Autodesk Inventor part; units mm, degrees
ref_plane "Work Plane1" through (25.5, 0, 0) normal (1, 0, 0) x (0, 0, -1)
ref_plane "Work Plane2" through (17.5, 0, 0) normal (-1, 0, 0) x (0, 0, 1)
ref_plane "YZ Plane" through (0, 0, 0) normal (1, 0, 0) x (0, 1, 0)
sketch "Sketch1" plane through (0, 0, 0) normal (1, 0, 0) x (0, 1, 0)
  circle A0 centre (0, 0) radius 2.85
  dimension "diameter" = 5.7
extrude "Shaft" add sketch "Sketch1" along normal mid plane 47
sketch "Sketch2" plane through (0, 0, 0) normal (0, 0, 1) x (1, 0, 0)
  line L0 (-23.5, -2.85) -> (-23.5, 2.85) construction
  line L1 (23.5, -2.85) -> (-23.5, -2.85) construction
  line L2 (23.5, 2.85) -> (23.5, -2.85) construction
  line L3 (-23.5, 2.85) -> (23.5, 2.85) construction
  line L4 (-23.5, -2.85) -> (23.5, -2.85)
  line L5 (-16.5, -2.85) -> (-16.5, -2.85)
  line L6 (-23.5, -2.85) -> (23.5, -2.85)
  line L7 (-21.5, 0) -> (-17.5, 0) construction
  line L8 (-20.6, -0.9) -> (-18.4, -0.9)
  line L9 (-18.4, 0.9) -> (-20.6, 0.9)
  arc A0 (-20.6, 0.9) -> (-20.6, -0.9) centre (-20.6, 0) ccw
  arc A1 (-18.4, -0.9) -> (-18.4, 0.9) centre (-18.4, 0) ccw
  point P0 (0, 0)
  point P1 (23.5, 0)
  point P2 (-19.5, 0)
  dimension "d17" = 1.8
  dimension "d20" = 2
  dimension "d21" = 1
  dimension "d22" = 7
extrude "Slot for Differential Gear" cut sketch "Sketch2" along normal through all both and the other way through all
ref_plane "Work Plane1" through (25.5, 0, 0) normal (1, 0, 0) x (0, 0, -1)
sketch "Sketch3" plane through (25.5, 0, 0) normal (1, 0, 0) x (0, 0, -1)
  arc A0 (1.6583, -2.5) -> (-1.6583, -2.5) centre (0, 0) ccw construction
  circle A1 centre (0, 0) radius 2.85 construction
  line L0 (-1.6583, -2.5) -> (1.6583, -2.5)
  arc A2 (1.6125, -2.35) -> (-1.6125, -2.35) centre (0, 0) ccw
  line L1 (1.6125, -2.35) -> (-1.6125, -2.35)
  point P0 (-1.3684, -2.5)
  point P1 (1.3684, -2.5)
  dimension "d49" = 3
  dimension "d50" = 2.5
  dimension "wheel_offset" = 0.15
extrude "Wheel Insert Profile" add sketch "Sketch3" along normal blind 12
loft "Loft1" add section 1 edges at (23.5, -2.85, 0) section 2 edges at (25.5, -2.35, 0) (25.5, 2.85, 0)
ref_plane "Work Plane2" through (17.5, 0, 0) normal (-1, 0, 0) x (0, 0, 1)
sketch "Sketch4" plane through (17.5, 0, 0) normal (-1, 0, 0) x (0, 0, 1)
  circle A0 centre (0, 0) radius 3.75
  dimension "d35" = 7.5
extrude "Stopper" add sketch "Sketch4" against normal blind 1
fillet "Fillet1" radius 0.5 2 edges at (17.5, 0, -3.75) (18.5, 0, -3.75)
sketch "Sketch8" plane through (-23.5, 0, 0) normal (-1, 0, 0) x (0, 0, 1)
  circle A0 centre (0, 0) radius 2.85
  circle A1 centre (0, 0) radius 2.7 construction
  circle A2 centre (0, 0) radius 2.65
  dimension "d68" = 5.4
  dimension "d69" = 0.05
extrude "Differential Gear Insert Profile" cut sketch "Sketch8" against normal blind 8
fillet "Fillet3" radius 1 1 edges at (-15.5, -2.85, 0)
chamfer "Chamfer4" distance 0.5 angle 45 2 edges at (-23.5, 0, -2.65) (37.5, 2.85, 0)
properties part number "rear shaft v2"
The listing builds one solid part. Answer for the finished solid, in the listing's coordinates (mm). A direction names the side the tool comes from. Round coordinates to 2 decimals unless told otherwise and drop trailing zeros. Write each loop counter-clockwise with the first axis right and the second up, starting at its lowest first coordinate (ties: lowest second). Pieces come first, ordered by that corner, then holes. Notation, with made-up numbers: M 87.5,25 L 103.5,25 A7 cw 103.5,29 Z; hole C 78.5,-37 d7. An arc over 180 degrees is marked long. Write each question's results on one line, items separated by ' | '. Start each with the question number.
(1) Determine the mould class of faces 1 (the cylindrical face through (-17.5, 0, 0)), 2 (the cylindrical face through (31.17, 2.85, 0.1)), 3 (the flat face through (-23.5, 0, 0)) for opening direction Y: +Y half, -Y half, draft (parallel to the pull), parting line (faces both ways), or undercut.
(2) Find the intervals of material crossed by line 1 (X direction, y = -0.25, z = -2.25); line 2 (X direction, y = 2.25, z = 2.5); line 3 (Z direction, x = 25, y = -0.25), in increasing order.
(3) Each of these flat-tipped pins is pushed along its axis until it touches: P1, Ø3, axis at x = -10, y = 0.5, coming from the +Z side; P2, Ø1.1, axis at x = -20, z = 1, coming from the -Y side; P3, Ø1, axis at x = 30.5, z = -1.5, coming from the +Y side. Where does it stop, or does it pass through?
(4) For faces 4 (the flat face through (31, -2.35, 0)), 5 (the flat face through (-19, 0.9, 0)), 6 (the cylindrical face through (-19.303, -2.351, 1.223)), determine the directions among +Z, -Z, +X, -X, +Y, -Y from which every point of the face is accessible in a straight line to the end or side of a thin tool.
(5) The part is cut by section A-A, the plane x = 14.5. Write down the section's boundary in (y, z), and give its area (3 significant figures).
Worked answers:
1) face 1: undercut | face 2: parting line | face 3: draft
2) line 1: x = -23.39 to -21.46, -17.54 to 37.5 | line 2: x = 17.51 to 18.49 | line 3: z = -2.84 to 2.84
3) P1: stops at z = 2.85 | P2: stops at y = -2.61 | P3: stops at y = 2.67
4) face 4: +Z, -Z, +X, -Y | face 5: +Z, -Z | face 6: -X
5) outline: C 0,0 d5.7 | area: 25.5 mm²
